The listing builds one solid part. Answer for the finished solid, in the listing's coordinates (mm). Round coordinates to 2 decimals unless told otherwise and drop trailing zeros. Loops run counter-clockwise (first coordinate to the right, second up) from the corner with the lowest first, then second, coordinate; pieces in that order, holes last. Notation, with made-up numbers: (-37, 1) -> (16, 1) arc R22 ccw to (16, 29) -> close; hole circle Ø1 at (-28, -14). An arc over 180 degrees is marked (long way). Write each question's results on one line, items separated by ' | '. Start each with the question number.
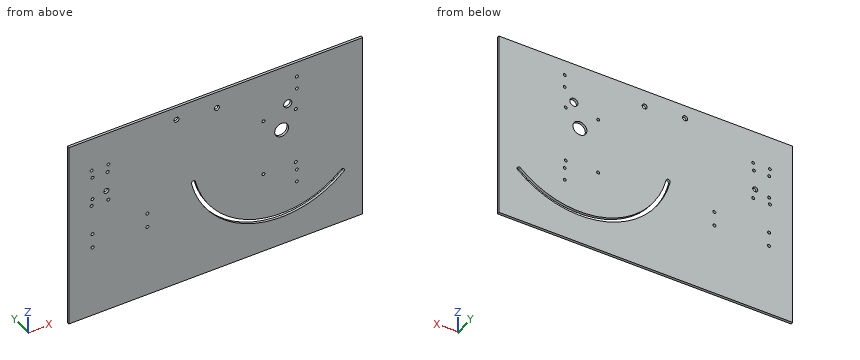
from build123d import *

# Parameters (mm, degrees)
SKETCH1_W           = 317.5
SKETCH1_H           = 177.8
SKETCH1_R           = 3.175
SKETCH1_R_2         = 8.73125
SKETCH1_R_3         = 1.905
BOSS_EXTRUDE1_DEPTH = 3.175
SKETCH3_R           = 3.175
CUT_EXTRUDE2_DEPTH  = 182.974869488
SKETCH4_W           = 25.4
SKETCH4_H           = 177.8
CUT_EXTRUDE3_DEPTH  = 182.974869488
SKETCH5_R           = 5.08
CUT_EXTRUDE4_DEPTH  = 182.974869488
SKETCH6_R           = 1.8034
CUT_EXTRUDE5_DEPTH  = 182.974869488
SKETCH7_R           = 1.8415
CUT_EXTRUDE6_DEPTH  = 182.974869488
BOSS_EXTRUDE2_DEPTH = 3.175
CUT_EXTRUDE7_DEPTH  = 256.444486386


with BuildPart() as part:
    # Sketch1 → Boss-Extrude1 (new body)
    with BuildSketch(Plane(origin=(0, 0, 0), x_dir=(1, 0, 0), z_dir=(0, 1, 0))):
        Rectangle(SKETCH1_W, SKETCH1_H)
        with Locations(Location((-111.76, -12.7, 0), (0, 0, 270))):
            Circle(SKETCH1_R, mode=Mode.SUBTRACT)
        with Locations(Location((107.95, -6.35, 0), (0, 0, 270))):
            Circle(SKETCH1_R_2, mode=Mode.SUBTRACT)
        with Locations(Location((-129.032, 55.88, 0), (0, 0, 270))):
            Circle(SKETCH1_R_3, mode=Mode.SUBTRACT)
        with Locations(Location((-60.452, 55.88, 0), (0, 0, 270))):
            Circle(SKETCH1_R_3, mode=Mode.SUBTRACT)
        with Locations(Location((-129.032, 38.1, 0), (0, 0, 270))):
            Circle(SKETCH1_R_3, mode=Mode.SUBTRACT)
        with Locations(Location((-60.452, 38.1, 0), (0, 0, 270))):
            Circle(SKETCH1_R_3, mode=Mode.SUBTRACT)
    extrude(amount=BOSS_EXTRUDE1_DEPTH)

    # Sketch3 → Cut-Extrude2 (cut, through all)
    with BuildSketch(Plane(origin=(0, 0, 0), x_dir=(-1, 0, 0), z_dir=(0, -1, 0))):
        with Locations(Location((23.829539609, -72.39, 0), (0, 0, 90))):
            Circle(SKETCH3_R)
        with Locations(Location((-26.764302072, -67.818, 0), (0, 0, 90))):
            Circle(SKETCH3_R)
    extrude(amount=-CUT_EXTRUDE2_DEPTH, mode=Mode.SUBTRACT)

    # Sketch4 → Cut-Extrude3 (cut, through all)
    with BuildSketch(Plane(origin=(0, 3.175, 0), x_dir=(1, 0, 0), z_dir=(0, 1, 0))):
        with Locations((146.05, 0)):
            Rectangle(SKETCH4_W, SKETCH4_H)
    extrude(amount=-CUT_EXTRUDE3_DEPTH, mode=Mode.SUBTRACT)

    # Sketch5 → Cut-Extrude4 (cut, through all)
    with BuildSketch(Plane(origin=(0, 3.175, 0), x_dir=(1, 0, 0), z_dir=(0, 1, 0))):
        with Locations(Location((115.57, -38.1, 0), (0, 0, 270))):
            Circle(SKETCH5_R)
    extrude(amount=-CUT_EXTRUDE4_DEPTH, mode=Mode.SUBTRACT)

    # Sketch6 → Cut-Extrude5 (cut, through all)
    with BuildSketch(Plane.XZ):
        with Locations(Location((127, 69.85, 0), (0, 0, 270))):
            Circle(SKETCH6_R)
        with Locations(Location((127, 53.975, 0), (0, 0, 270))):
            Circle(SKETCH6_R)
        with Locations(Location((127, -53.975, 0), (0, 0, 270))):
            Circle(SKETCH6_R)
        with Locations(Location((127, -69.85, 0), (0, 0, 270))):
            Circle(SKETCH6_R)
    extrude(amount=-CUT_EXTRUDE5_DEPTH, mode=Mode.SUBTRACT)

    # Sketch7 → Cut-Extrude6 (cut, through all)
    with BuildSketch(Plane(origin=(0, 3.175, 0), x_dir=(1, 0, 0), z_dir=(0, 1, 0))):
        with Locations(Location((125.73, 43.4975, 0), (0, 0, 270))):
            Circle(SKETCH7_R)
        with Locations(Location((85.09, 43.4975, 0), (0, 0, 270))):
            Circle(SKETCH7_R)
        with Locations(Location((85.09, -26.9875, 0), (0, 0, 270))):
            Circle(SKETCH7_R)
        with Locations(Location((125.73, -26.9875, 0), (0, 0, 270))):
            Circle(SKETCH7_R)
        with Locations(Location((-130.175, -46.99, 0), (0, 0, 270))):
            Circle(SKETCH7_R)
        with Locations(Location((-109.22, -46.99, 0), (0, 0, 270))):
            Circle(SKETCH7_R)
        with Locations(Location((-129.2225, -37.1475, 0), (0, 0, 270))):
            Circle(SKETCH7_R)
        with Locations(Location((-110.1725, -37.1475, 0), (0, 0, 270))):
            Circle(SKETCH7_R)
        with Locations(Location((-129.2225, -8.5725, 0), (0, 0, 270))):
            Circle(SKETCH7_R)
        with Locations(Location((-130.175, 0, 0), (0, 0, 270))):
            Circle(SKETCH7_R)
        with Locations(Location((-109.22, 0, 0), (0, 0, 270))):
            Circle(SKETCH7_R)
    extrude(amount=-CUT_EXTRUDE6_DEPTH, mode=Mode.SUBTRACT)

    # Sketch8 → Boss-Extrude2 (add, through all)
    with BuildSketch(Plane.XZ):
        Polygon((133.35, 88.9), (133.35, -88.9), (-158.75, -88.9), (-158.75, -146.05), (209.55, -146.05), (209.55, 88.9), align=None)
    extrude(amount=-BOSS_EXTRUDE2_DEPTH)

    # Sketch9 → Cut-Extrude7 (cut, through all)
    with BuildSketch(Plane.XZ):
        with BuildLine():
            ThreePointArc((185.852793296, -79.875035933), (186.034700239, -76.287542398), (182.447206704, -76.105635455))
            ThreePointArc((182.447206704, -76.105635455), (74.993781285, -99.775648516), (-0.149958886, -19.401980777))
            ThreePointArc((-0.149958886, -19.401980777), (-3.209431792, -17.519741277), (-5.091671292, -20.579214184))
            ThreePointArc((-5.091671292, -20.579214184), (73.487211286, -104.627106734), (185.852793296, -79.875035933))
        make_face()
    extrude(amount=-CUT_EXTRUDE7_DEPTH, mode=Mode.SUBTRACT)


solid = part.part
Item 1: The part is cut by section A-A, the plane x = 17.5. Give the vertices of the cut face in (y, z) (3 decimals), plus the area to 3 significant figures.
Item 2: The part is cut by section D-D, the plane x = 155.5. Give the vertices of the cut face in (y, z) (3 decimals).
Item 3: Straight lines are drawn through the part: L1, parallel to X at y = 2.25, z = 6.35; L2, parallel to X at y = 2.1, z = 12.7 (3 decimals); L3, parallel to X at y = 2.1, z = -70. For each, find the intervals that lie inside material, in ascending order. Write a range as [from, to].
Item 4: The part is cut by section B-B, the plane z = -95. Give the number of separate pieces and of enclosed holes in the cut face, plus the area to 3 significant figures.
Report:
1) outline: (0, -146.05) -> (3.175, -146.05) -> (3.175, -66.605) -> (0, -66.605) -> close; (0, -58.207) -> (3.175, -58.207) -> (3.175, 88.9) -> (0, 88.9) -> close | area: 719 mm2
2) outline: (0, -146.05) -> (3.175, -146.05) -> (3.175, -99.681) -> (0, -99.681) -> close; (0, -94.088) -> (3.175, -94.088) -> (3.175, 88.9) -> (0, 88.9) -> close
3) L1: x = [-158.75, 99.22], [116.68, 209.55] | L2: x = [-158.75, -114.935], [-108.585, 101.957], [113.943, 209.55] | L3: x = [-158.75, 20.35], [27.21, 125.2], [128.8, 209.55]
4) separate pieces: 3 | enclosed holes: 0 | area: 1,100 mm2
